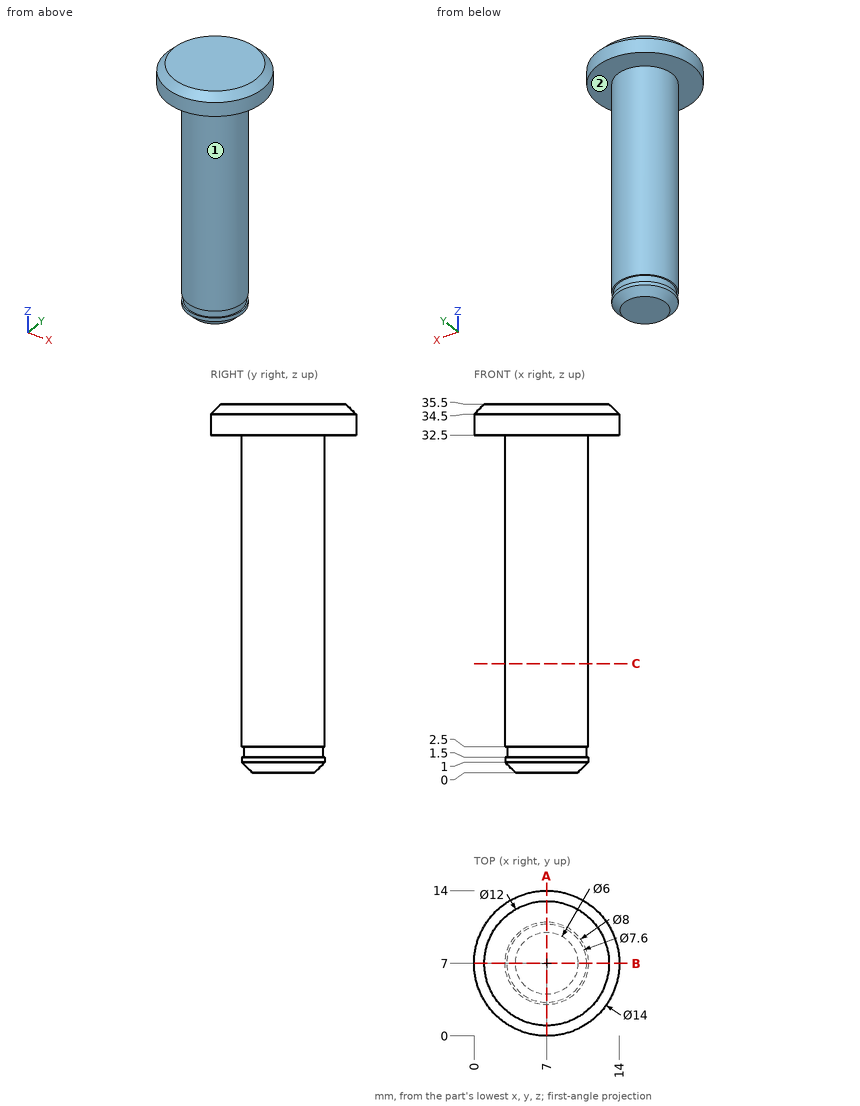
Check sheet for the drawn part. Datum: minimum x, y, z corner. Units: mm. Give positions to 0.01 mm unless a question says otherwise; leave off trailing zeros. Order: outer loops, then holes, each group sorted by start corner. A loop starts at its lowest first (then second) coordinate and runs counter-clockwise, first axis right, second up.
1. Depth check by flat-ended pin: pin 1 (4 mm diameter, centred on y = 6.5, z = 8.5, fed in from -X); pin 2 (2 mm diameter, centred on y = 11, z = 6.5, fed in from +X); pin 3 (3 mm diameter, centred on x = 8.5, z = 16.5, fed in from +Y). Enter the tip coordinate at first touch or a pass-through.
Completed:
pin 1: stops at x = 3
pin 2: stops at x = 9.65
pin 3: stops at y = 11
2. Sectioned sample at C-C (z = 10.5). Record the boundary of the cut face in (x, y), then the cut area to 3 significant figures.
Completed:
outline: circle Ø8 at (7, 7)
area: 50.3 mm2
3. Draft check along X on the marked faces 1 and 2. Enter one of: pulls with the +X half, pulls with the -X half, needs draft (parallel to the pull), parting line crosses it, or undercut.
Completed:
face 1: parting line crosses it
face 2: needs draft
4. Sectioned sample at A-A (x = 7). Record the boundary of the cut face in (y, z), then the cut area to 3 significant figures.
Completed:
outline: (0, 32.5) - (3, 32.5) - (3, 2.5) - (3.2, 2.5) - (3.2, 1.5) - (3, 1.5) - (3, 1) - (4, 0) - (10, 0) - (11, 1) - (11, 1.5) - (10.8, 1.5) - (10.8, 2.5) - (11, 2.5) - (11, 32.5) - (14, 32.5) - (14, 34.5) - (13, 35.5) - (1, 35.5) - (0, 34.5) - close
area: 300 mm2
5. Scan lines: line 1 (Z direction, x = 4, y = 9.5); line 2 (X direction, y = 5.75, z = 23.5); line 3 (Z direction, x = 3, y = 3). Record each from-to range of solid material in increasing order.
Completed:
line 1: z = 0.91 to 1.5, 2.5 to 35.5
line 2: x = 3.2 to 10.8
line 3: z = 32.5 to 35.5
